Geometry: see drawing. Coordinates: mm, zero at the bounding-box minimum. A direction names the side the tool comes from. Coordinates: 2 decimals unless noted, no trailing zeros. Loops run counter-clockwise (first coordinate to the right, second up) from the corner with the lowest first, then second, coordinate; pieces in that order, holes last. Notation, with made-up numbers: (53.25, 36) -> (108.25, 36) arc R9 cw to (108.25, 48) -> close; hole circle Ø1 at (12.25, 3.25). An arc over 180 degrees is marked (long way). Answer as a JSON object with one key per item and string values.
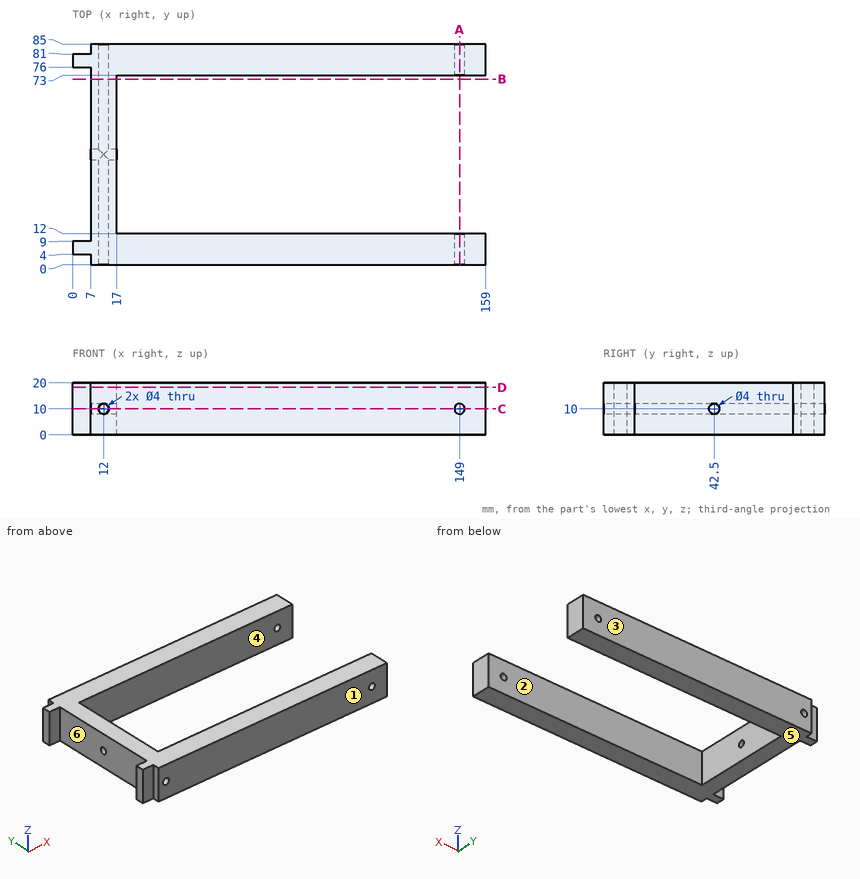
1. Section query A-A (x = 149). Return loops of the section in (y, z).
Reply:
{"outline": "(0, 0) -> (12, 0) -> (12, 8) -> (0, 8) -> close; (0, 12) -> (12, 12) -> (12, 20) -> (0, 20) -> close; (73, 0) -> (85, 0) -> (85, 8) -> (73, 8) -> close; (73, 12) -> (85, 12) -> (85, 20) -> (73, 20) -> close"}
2. Access query for the marked faces 1 and 2. Directions: +Z, -Z, +X, -X, +Y, -Y. A direction counts if a zero-diameter tool reaches every point of the face in a straight line with its end or side. Return the directions, or none.
Reply:
{"face 1": "+Z, -Z, +X, -X, -Y", "face 2": "+Z, -Z, +X"}
3. Line query: line 1 along Y through (x, z) = (128.5, 17); line 2 along Z through (x, y) = (12, 74); line 3 along Y through (x, z) = (9.55, 10). Output: solid intervals per line, ascending.
Reply:
{"line 1": "y = 0 to 12, 73 to 85", "line 2": "z = 0 to 8, 12 to 20", "line 3": "y = 0 to 40.5, 44.5 to 85"}
4. Pin query (flat end, axial travel): P1, Ø6, axis at y = 27, z = 18, coming from the -X side; P2, Ø4.5, axis at x = 149, z = 10, coming from the +Y side; P3, Ø7.5, axis at x = 3, z = 6.5, coming from the -Y side; P4, Ø1.5, axis at y = 14, z = 17.5, coming from the +X side. Return the tip coordinate at first contact, or that it passes through.
Reply:
{"P1": "stops at x = 7", "P2": "stops at y = 85", "P3": "stops at y = 4", "P4": "stops at x = 17"}
5. Section query C-C (z = 10). Count the separate pieces of the cut face and the enclosed holes in it, plus the area to 3 significant figures.
Reply:
{"separate pieces": "6", "enclosed holes": "0", "area": "3,870 mm2"}
6. Section query D-D (z = 18.25). Return loops of the section in (x, y), plus the area to 3 significant figures.
Reply:
{"outline": "(0, 4) -> (7, 4) -> (7, 0) -> (159, 0) -> (159, 12) -> (17, 12) -> (17, 73) -> (159, 73) -> (159, 85) -> (7, 85) -> (7, 81) -> (0, 81) -> (0, 76) -> (7, 76) -> (7, 9) -> (0, 9) -> close", "area": "4,330 mm2"}
7. Section query B-B (y = 71.5). Return loops of the section in (x, z).
Reply:
{"outline": "(7, 0) -> (17, 0) -> (17, 20) -> (7, 20) -> close; hole circle Ø4 at (12, 10)"}
8. Mould query, pull axis Y, two halves, no side actions, for the marked faces 3, 4, 5 and 6. Classes: pulls with the +Y half, pulls with the -Y half, needs draft (parallel to the pull), parting line crosses it, or undercut.
Reply:
{"face 3": "pulls with the +Y half", "face 4": "undercut", "face 5": "needs draft", "face 6": "undercut"}
